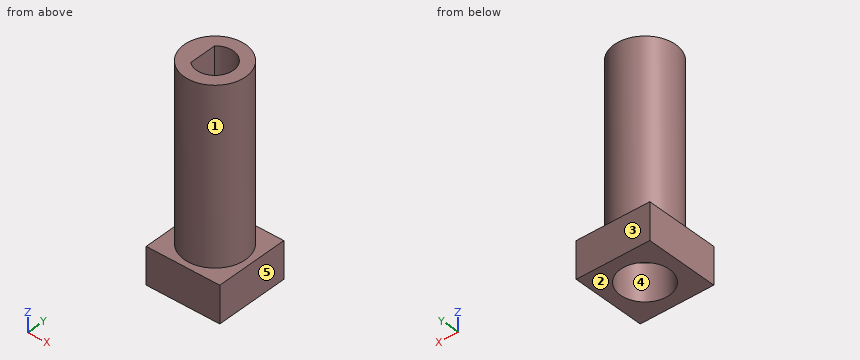
```python
from build123d import *

# Parameters (mm, degrees)
SKETCH1_W           = 12
SKETCH1_H           = 12
BOSS_EXTRUDE1_DEPTH = 6
SKETCH2_R           = 5
BOSS_EXTRUDE2_DEPTH = 10
SKETCH3_R           = 5
BOSS_EXTRUDE3_DEPTH = 18.3
CUT_EXTRUDE2_DEPTH  = 22
SKETCH6_R           = 4
CUT_EXTRUDE3_DEPTH  = 6


with BuildPart() as part:
    # Sketch1 → Boss-Extrude1 (new body)
    with BuildSketch(Plane.XY):
        Rectangle(SKETCH1_W, SKETCH1_H)
    extrude(amount=BOSS_EXTRUDE1_DEPTH)

    # Sketch2 → Boss-Extrude2 (add)
    with BuildSketch(Plane.XY.offset(6)):
        Circle(SKETCH2_R)
    extrude(amount=BOSS_EXTRUDE2_DEPTH)

    # Sketch3 → Boss-Extrude3 (add)
    with BuildSketch(Plane.XY.offset(16)):
        Circle(SKETCH3_R)
    extrude(amount=BOSS_EXTRUDE3_DEPTH)

    # Sketch5 → Cut-Extrude2 (cut)
    with BuildSketch(Plane.XY.offset(34.3)):
        with BuildLine():
            Line((-2, 2.236067977), (-2, -2.236067977))
            ThreePointArc((-2, -2.236067977), (3, 0), (-2, 2.236067977))
        make_face()
    extrude(amount=-CUT_EXTRUDE2_DEPTH, mode=Mode.SUBTRACT)

    # Sketch6 → Cut-Extrude3 (cut)
    with BuildSketch(Plane(origin=(0, 0, 0), x_dir=(-1, 0, 0), z_dir=(0, 0, -1))):
        Circle(SKETCH6_R)
    extrude(amount=-CUT_EXTRUDE3_DEPTH, mode=Mode.SUBTRACT)


solid = part.part
```
Check sheet for the modelled part. Datum: model origin and axes. Units: mm. Face numbers are marked on the shaded views. A direction names the side the tool comes from. Round coordinates to 2 decimals unless told otherwise and drop trailing zeros. Loops run counter-clockwise (first coordinate to the right, second up) from the corner with the lowest first, then second, coordinate; pieces in that order, holes last. Notation, with made-up numbers: M -36,88 L -12,88 A22 ccw -12,106 Z; hole C -28,24 d1. An arc over 180 degrees is marked long. Answer as a JSON object with one key per item and string values.
1. Mould release check, pull along Y, two halves, no side actions. Record for the marked faces 3, 4 and 5: pulls with the +Y half, pulls with the -Y half, needs draft (parallel to the pull), parting line crosses it, or undercut.
Reply:
{"face 3": "pulls with the +Y half", "face 4": "undercut", "face 5": "needs draft"}
2. Section check C-C (z = 17). Record the boundary of the cut face in (x, y).
Reply:
{"outline": "C 0,0 d10; hole M -2,-2.24 A3 ccw long -2,2.24 Z"}
3. Section check D-D (z = 11.5). Record the boundary of the cut face in (x, y).
Reply:
{"outline": "C 0,0 d10"}
4. Gauge pin test, flat ends, axial feed: P1, Ø6, axis at y = 1, z = 7, coming from the -X side; P2, Ø3.5, axis at x = 0, y = 0, coming from the -Z side; P3, Ø1, axis at x = 3, z = 27.5, coming from the -Y side; P4, Ø1.5, axis at x = 0, y = 0, coming from the +Z side. Record the tip position at first contact, or that the pin passes through.
Reply:
{"P1": "stops at x = -6", "P2": "stops at z = 6", "P3": "stops at y = -4.33", "P4": "stops at z = 12.3"}
5. Section check B-B (y = 1.25). Record the boundary of the cut face in (x, z).
Reply:
{"outline": "M -6,0 L -3.8,0 L -3.8,6 L 3.8,6 L 3.8,0 L 6,0 L 6,6 L 4.84,6 L 4.84,34.3 L 2.73,34.3 L 2.73,12.3 L -2,12.3 L -2,34.3 L -4.84,34.3 L -4.84,6 L -6,6 Z"}
6. Section check A-A (x = 0). Record the boundary of the cut face in (y, z).
Reply:
{"outline": "M -6,0 L -4,0 L -4,6 L 4,6 L 4,0 L 6,0 L 6,6 L 5,6 L 5,34.3 L 3,34.3 L 3,12.3 L -3,12.3 L -3,34.3 L -5,34.3 L -5,6 L -6,6 Z"}
7. Access from +Z, -Z, +X, -X, +Y, -Y to the whole of each face (thin tool, end or side, straight path). Record for the marked faces 1 and 2.
Reply:
{"face 1": "+Z", "face 2": "-Z, +X, -X, +Y, -Y"}
8. Scan lines: line 1 (Y direction, x = 0, z = 4.1); line 2 (Y direction, x = 0, z = 22.25); line 3 (Z direction, x = -1.75, y = -1.5). Record each from-to range of solid material in increasing order.
Reply:
{"line 1": "y = -6 to -4, 4 to 6", "line 2": "y = -5 to -3, 3 to 5", "line 3": "z = 6 to 12.3"}
